from build123d import *

# Parameters (mm, degrees)
SKETCH058_W  = 10
SKETCH058_H  = 3
PAD058_DEPTH = 3
FILLET_R     = 0.5
FILLET001_R  = 0.5
SKETCH057_R  = 2.5
PAD057_DEPTH = 4
SKETCH056_R  = 22.5
PAD056_DEPTH = 6.35


with BuildPart() as fillet001:
    # Sketch058 → Pad058 (new body)
    with BuildSketch(Plane.XZ):
        with Locations((5, -1.5)):
            Rectangle(SKETCH058_W, SKETCH058_H)
    extrude(amount=PAD058_DEPTH)

    # Fillet
    fillet_edges = [fillet001.edges().sort_by_distance(p)[0] for p in [
        (10, -1.5, -3),
    ]]
    fillet(fillet_edges, radius=FILLET_R)

    # Fillet001
    fillet001_edges = [fillet001.edges().sort_by_distance(p)[0] for p in [
        (10, -1.5, 0),
    ]]
    fillet(fillet001_edges, radius=FILLET001_R)


with BuildPart() as fillet001_1:
    # Fillet001 placement: moved
    add(fillet001.part.moved(Location((-23, 0, 0))))


with BuildPart() as body057:
    # Sketch057 → Pad057 (new body)
    with BuildSketch(Plane.XZ):
        Circle(SKETCH057_R)
    extrude(amount=PAD057_DEPTH)


with BuildPart() as body057_1:
    # Body057 placement: moved
    add(body057.part.moved(Location((10, 0, -10))))


with BuildPart() as ledplate:
    # Sketch056 → Pad056 (new body)
    with BuildSketch(Plane.XZ):
        Circle(SKETCH056_R)
    extrude(amount=PAD056_DEPTH)

    # Cut061: cut Body057
    add(body057_1.part, mode=Mode.SUBTRACT)

    # Cut062: cut Fillet001
    add(fillet001_1.part, mode=Mode.SUBTRACT)


with BuildPart() as ledplate_1:
    # Cut062 placement: moved
    add(ledplate.part.moved(Location((0, 14.75, 0))))


solid = ledplate_1.part
Build history of the part. All positions in model axes, mm. A direction names the side the tool comes from. Give positions to 0.01 mm unless a question says otherwise; leave off trailing zeros. Order: outer loops, then holes, each group sorted by start corner. A loop starts at its lowest first (then second) coordinate and runs counter-clockwise, first axis right, second up. Notation, with made-up numbers: M 28.5,-16.75 L 54.5,-16.75 A26 ccw 54.5,22.25 Z; hole C 73,40 d4. An arc over 180 degrees is marked long. Put each result on its own line as item: value.
Item 1: Probe line 1 (Z direction, x = 10, y = 13.4); line 2 (X direction, y = 12.75, z = -9); line 3 (Y direction, x = 8.5, z = -10). List the from-to ranges inside material, lowest first. Write a range as [from, to].
From the geometry:
line 1: z = [-20.16, -12.5], [-7.5, 20.16]
line 2: x = [-20.62, 7.71], [12.29, 20.62]
line 3: y = [8.4, 10.75]
Item 2: Slice it at C-C, the plane x = 10. Write the cut outline in (y, z).
From the geometry:
outline: M 8.4,-20.16 L 14.75,-20.16 L 14.75,-12.5 L 10.75,-12.5 L 10.75,-7.5 L 14.75,-7.5 L 14.75,20.16 L 8.4,20.16 Z
Item 3: Slice it at D-D, the plane z = -6. Write the cut outline in (x, y).
From the geometry:
outline: M -21.69,8.4 L 21.69,8.4 L 21.69,14.75 L -21.69,14.75 Z
Item 4: Two-plate mould, pull along Z, no slides. Class faces 1 (the cylindrical face through (9.46, 12.78, -12.44)), 2 (the cylindrical face through (10.382, 11.619, -19.961)), 3 (the flat face through (-18, 13, 0)), 4 (the flat face through (0, 14.75, 0)): +Z half, -Z half, draft (parallel to the pull), parting line (faces both ways), or undercut.
From the geometry:
face 1: undercut
face 2: parting line
face 3: undercut
face 4: draft
Item 5: Slice it at A-A, the plane y = 12.75. Write the cut outline in (x, z).
From the geometry:
outline: M -22.5,0 L -13.5,0 A0.5 cw -13,-0.5 L -13,-2.5 A0.5 cw -13.5,-3 L -22.3,-3 A22.5 ccw long Z; hole C 10,-10 d5
Item 6: 3-axis set-ups, long thin cutter, end or side, ignore diameter. For faces 5 (the flat face through (-13, 13, -2)), 6 (the flat face through (0, 8.4, 0)), 7 (the flat face through (10, 10.75, -10)): which of +Z, -Z, +X, -X, +Y, -Y reach the whole face in a straight line?
From the geometry:
face 5: -X, +Y
face 6: +Z, -Z, +X, -X, -Y
face 7: +Y
Item 7: Flat gauge pins, fed straight in: pin 1 Ø3 at (y, z) = (13.5, 14) entering from +X; pin 2 Ø3 at (x, y) = (-3, 13) entering from -Z; pin 3 Ø2 at (y, z) = (13, -1.5) entering from -X. Where does each tip first touch, or does it go through?
From the geometry:
pin 1: stops at x = 18.71
pin 2: stops at z = -22.45
pin 3: stops at x = -13
Item 8: Slice it at B-B, the plane z = -11. Write the cut outline in (x, y).
From the geometry:
outline: M -19.63,8.4 L 19.63,8.4 L 19.63,14.75 L 12.29,14.75 L 12.29,10.75 L 7.71,10.75 L 7.71,14.75 L -19.63,14.75 Z
